Design review of the part built by this model. Coordinates are the model's own, in mm. A direction names the side the tool comes from. Give positions to 0.01 mm unless a question says otherwise; leave off trailing zeros. Loops run counter-clockwise (first coordinate to the right, second up) from the corner with the lowest first, then second, coordinate; pieces in that order, holes last. Notation, with made-up numbers: (41.5, -40) -> (83.5, -40) arc R23 ccw to (83.5, -29) -> close; hole circle Ø9 at (88.25, 34). An arc over 180 degrees is marked (long way). Answer as CSV lines item,"result".
from build123d import *

# Parameters (mm, degrees)
BOSS_EXTRUDE1_DEPTH = 5.715
SKETCH2_R           = 2.794
BOSS_EXTRUDE3_DEPTH = 2.8575


with BuildPart() as part:
    # Sketch1 → Boss-Extrude1 (new body)
    with BuildSketch(Plane(origin=(0, 0, 0), x_dir=(1, 0, 0), z_dir=(0, 1, 0))):
        Polygon((-5.674598366, 20.311212687), (7.025401634, 20.311212687), (7.025401634, 7.611212687), (19.725401634, 7.611212687), (19.725401634, -17.788787313), (7.025401634, -17.788787313), (7.025401634, -5.088787313), (-5.674598366, -5.088787313), align=None)
    extrude(amount=BOSS_EXTRUDE1_DEPTH)

    # Sketch2 → Boss-Extrude3 (add)
    with BuildSketch(Plane(origin=(0, 5.715, 0), x_dir=(1, 0, 0), z_dir=(0, 1, 0))):
        with Locations(Location((0.675401634, 1.261212687, 0), (0, 0, 90))):
            Circle(SKETCH2_R)
        with Locations(Location((13.375401634, 1.261212687, 0), (0, 0, 90))):
            Circle(SKETCH2_R)
        with Locations(Location((0.675401634, 13.961212687, 0), (0, 0, 90))):
            Circle(SKETCH2_R)
        with Locations(Location((13.375401634, -11.438787313, 0), (0, 0, 90))):
            Circle(SKETCH2_R)
    extrude(amount=BOSS_EXTRUDE3_DEPTH)


solid = part.part
Q1. We need section D-D, the plane y = 7.75. State the section outline as (x, z) points.
Filled sheet:
outline,"circle Ø5.59 at (0.68, -13.96); circle Ø5.59 at (0.68, -1.26); circle Ø5.59 at (13.38, -1.26); circle Ø5.59 at (13.38, 11.44)"
Q2. For faces 4 (the flat face through (13, 3, -7.611)), 5 (the flat face through (7.025, 3, 12)), 6 (the cylindrical face through (-0.164, 7.124, -3.926)), 7 (the flat face through (1, 8.572, -14)), list the 3-axis set-ups (+Z, -Z, +X, -X, +Y, -Y) from which the entire face can be reached by the end or side of a thin tool; tool diameter is ignored.
Filled sheet:
face 4,"-Z, +X, +Y, -Y"
face 5,"+Z, -X, +Y, -Y"
face 6,"+Y"
face 7,"+Z, -Z, +X, -X, +Y"
Q3. The part is to be moulded in two halves that separate along X. For faces 1 (the flat face through (7.025, 3, -14)), 2 (the cylindrical face through (16.103, 7.124, -0.656)), 3 (the flat face through (1, 3, -20.311)), say which applies: pulls with the +X half, pulls with the -X half, needs draft (parallel to the pull), parting line crosses it, or undercut.
Filled sheet:
face 1,"pulls with the +X half"
face 2,"undercut"
face 3,"needs draft"
Q4. We need section C-C, the plane x = 9.75. State the section outline as (y, z) points (3 decimals), and give its area (3 significant figures).
Filled sheet:
outline,"(0, -7.611) -> (5.715, -7.611) -> (5.715, 17.789) -> (0, 17.789) -> close"
area,"145 mm^2"
Q5. To check wall thickness, follow probe 1 along Y at (x, z) = (18.25, 8) (3 decimals); probe 2 along X at (y, z) = (2.5, 7.5); probe 3 along X at (y, z) = (8.25, -3). State the ranges of each line that lie inside material, in increasing order. Write a range as from..to.
Filled sheet:
probe 1,"y = 0..5.715"
probe 2,"x = 7.03..19.73"
probe 3,"x = -1.51..2.86, 11.19..15.56"
Q6. We need section A-A, the plane y = 5. State the section outline as (x, z) points, and give its area (3 significant figures).
Filled sheet:
outline,"(-5.67, -20.31) -> (7.03, -20.31) -> (7.03, -7.61) -> (19.73, -7.61) -> (19.73, 17.79) -> (7.03, 17.79) -> (7.03, 5.09) -> (-5.67, 5.09) -> close"
area,"645 mm^2"
Q7. Clearance check with flat-ended pins moving along their axes: pin 1 Ø3 at (x, y) = (1.5, 2) entering from +Z; pin 2 Ø1.5 at (y, z) = (6.5, 11) entering from -X; pin 3 Ø2 at (x, z) = (5, -13.5) entering from +Y (3 decimals). State where each tip first meets the part, or that it passes through.
Filled sheet:
pin 1,"stops at z = 5.09"
pin 2,"stops at x = 10.58"
pin 3,"stops at y = 5.715"
Q8. We need section B-B, the plane z = -15.5. State the section outline as (x, y) points (1 decimal), and give its area (3 significant figures).
Filled sheet:
outline,"(-5.7, 0) -> (7, 0) -> (7, 5.7) -> (3, 5.7) -> (3, 8.6) -> (-1.7, 8.6) -> (-1.7, 5.7) -> (-5.7, 5.7) -> close"
area,"85.9 mm^2"
